Autodesk Inventor part; units mm, degrees
ref_plane "YZ Plane" through (0, 0, 0) normal (1, 0, 0) x (0, 1, 0)
ref_plane "XZ Plane" through (0, 0, 0) normal (0, 1, 0) x (-1, 0, 0)
ref_plane "XY Plane" through (0, 0, 0) normal (0, 0, 1) x (1, 0, 0)
sketch "Sketch1" plane through (0, 0, 0) normal (0, 0, 1) x (1, 0, 0)
  line L0 (0, 0) -> (161.978778, 0)
  line L1 (161.978778, -12.7) -> (0, -12.7)
  line L2 (0, 0) -> (35.7378, 0)
  line L3 (35.7378, 0) -> (35.7378, -1.5875)
  line L4 (35.7378, -1.5875) -> (36.53155, -1.5875)
  line L5 (36.53155, -1.5875) -> (36.53155, 0)
  line L6 (35.7378, -1.5875) -> (34.94405, -1.5875)
  line L7 (34.94405, -1.5875) -> (34.94405, 0)
  line L8 (36.53155, -12.7) -> (34.94405, -12.7)
  line L9 (34.94405, -12.7) -> (34.94405, -11.1125)
  line L10 (34.94405, -11.1125) -> (36.53155, -11.1125)
  line L11 (36.53155, -11.1125) -> (36.53155, -12.7)
  line L12 (161.978778, 0) -> (151.640978, 0)
sketch "Sketch3" plane through (0, 0, 0) normal (0, 0, -1) x (-1, 0, 0)
  circle A0 centre (6.35164, 38.1) radius 3.3782
  circle A1 centre (6.35164, 22.225) radius 3.3782
sketch "Sketch6" plane through (-12.7, 33.655, 84.38515) normal (0, 0, 1) x (1, 0, 0)
  line L0 (0, 0) -> (12.7, 0)
  line L1 (0, -33.655) -> (0, 0)
  line L2 (6.35, 0) -> (6.35, -11.218333)
  line L3 (6.35, -11.218333) -> (6.35, -22.445133)
  circle A0 centre (6.35, -11.218333) radius 3.3782
  circle A1 centre (6.35, -22.445133) radius 3.3782
  dimension "d29" = 11.21833
  dimension "d31" = 11.2268
  dimension "d32" = 6.7564
  dimension "d33" = 6.7564
sketch "Sketch1 outline for Plate1" plane through (0, 0, 0) normal (0, 0, 1) x (1, 0, 0)
  line L0 (0, 0) -> (-12.7, 0)
  line L1 (-12.7, 0) -> (-12.7, 44.45)
  line L2 (-12.7, 44.45) -> (0, 44.45)
  line L3 (0, 44.45) -> (0, 0)
extrude "Plate1" add sketch "Sketch1 outline for Plate1" along normal blind 3.175
sketch "Sketch2" plane through (0, -12.7, 0) normal (0, 0, 1) x (1, 0, 0)
  line L0 (35.7378, 11.1125) -> (35.7378, 12.7)
  line L1 (0, 12.7) -> (35.7378, 12.7)
  line L2 (36.53155, 12.7) -> (161.978778, 12.7)
  line L3 (35.7378, 11.1125) -> (34.94405, 11.1125)
  line L4 (34.94405, 11.1125) -> (34.94405, 12.7)
edge flange "Flange1" height 79.94015 angle 90 thickness 3.175 bend radius 1.27 thickness toward (0, -1, 0) relief straight relief width 3.175 relief depth 1.5875 edges at (-6.35, 0, 3.175) wall of the first edge with corners at (-12.7, -1.27, 4.445) (0, -1.27, 4.445) (0, -1.27, 79.94015) (-12.7, -1.27, 79.94015)
bend "Bend1"
corner "Corner1"
sketch "Sketch4" plane through (0, -12.7, 0) normal (0, 0, 1) x (1, 0, 0)
  line L0 (161.978778, 0) -> (36.53155, 0)
  line L1 (36.53155, 12.7) -> (161.978778, 12.7)
  line L2 (161.978778, 12.7) -> (115.445978, 12.7)
  line L3 (115.445978, 12.7) -> (115.445978, 11.1125)
  line L4 (115.445978, 11.1125) -> (116.239728, 11.1125)
  line L5 (116.239728, 11.1125) -> (116.239728, 12.7)
  line L6 (115.445978, 11.1125) -> (114.652228, 11.1125)
  line L7 (114.652228, 11.1125) -> (114.652228, 12.7)
  line L8 (140.845978, 0) -> (141.639728, 0)
  line L9 (141.639728, 0) -> (141.639728, 1.5875)
  line L10 (141.639728, 1.5875) -> (140.052228, 1.5875)
  line L11 (140.052228, 1.5875) -> (140.052228, 0)
  dimension "d15" = 1.5875
extrude "Cut1" cut sketch "Sketch3" against normal blind 3.175
sketch "Sketch5" plane through (0, -12.7, 0) normal (0, 0, 1) x (1, 0, 0)
  line L0 (115.445978, 12.7) -> (115.445978, 11.1125)
  line L1 (115.445978, 12.7) -> (161.978778, 12.7)
  line L2 (115.445978, 11.1125) -> (116.239728, 11.1125)
  line L3 (116.239728, 11.1125) -> (116.239728, 12.7)
edge flange "Flange2" height 38.1 angle 90 thickness 3.175 bend radius 1.27 thickness toward (0, 0, 1) relief straight relief width 3.175 relief depth 1.5875 edges at (-6.35, -1.27, 79.94015) wall of the first edge with corners at (-12.7, 0, 81.21015) (0, 0, 81.21015) (0, 33.655, 81.21015) (-12.7, 33.655, 81.21015)
bend "Bend2"
corner "Corner2"
extrude "Cut3" cut sketch "Sketch6" against normal blind 3.175
equation "\"d3\" = BendReliefWidth"
equation "\"d4\" = BendReliefDepth"
equation "\"d5\" = MinimumRemnant"
equation "\"d6\" = BendRadius"
equation "\"d10\" = CornerReliefSize"
equation "\"d11\" = GapSize"
equation "\"d12\" = JacobiRadiusSize"
equation "\"d19\" = BendReliefWidth"
equation "\"d20\" = BendReliefDepth"
equation "\"d21\" = MinimumRemnant"
equation "\"d22\" = BendRadius"
equation "\"d26\" = CornerReliefSize"
equation "\"d27\" = GapSize"
equation "\"d28\" = JacobiRadiusSize"
equation "\"BendRadius\" = Thickness"
equation "\"BendReliefWidth\" = Thickness"
equation "\"BendReliefDepth\" = 0.5 * Thickness"
equation "\"CornerReliefSize\" = 4 * Thickness"
equation "\"MinimumRemnant\" = 2 * Thickness"
equation "\"TransitionRadius\" = BendRadius"
equation "\"JacobiRadiusSize\" = Thickness"
equation "\"GapSize\" = Thickness"
equation "\"d2\" = BendRadius"
equation "\"d6\" = Thickness"
equation "\"d16\" = Thickness"
properties part number "M - bottom pulley mount v2" material "Aluminum 6061"
Read the model definition and answer for the solid it produces. Units are mm, in the model's axes. A direction names the side the tool comes from. Coordinates: 2 decimals unless noted, no trailing zeros. Order: outer loops, then holes, each group sorted by start corner. A loop starts at its lowest first (then second) coordinate and runs counter-clockwise, first axis right, second up. Notation, with made-up numbers: (-23.75, 66.5) - (-13.75, 66.5) arc R21 ccw to (-13.75, 98.5) - close; hole circle Ø7 at (24.5, 1). An arc over 180 degrees is marked (long way). Answer as a JSON object with one key per item and string values. Group by question number.
Item 1: Flat-ended cylindrical pins translate along their axes: P1, Ø5.5, axis at x = -6.35, y = 38.1, coming from the -Z side; P2, Ø3, axis at x = -8.5, z = 16.5, coming from the +Y side; P3, Ø1.6, axis at x = -4, z = 83, coming from the +Y side (3 decimals). Find the tip coordinate at first contact, or state that the pin passes through.
Item 2: Section A-A (x = -6.35) is taken. Give the vertices of the cut face in (y, z) (3 decimals), plus the area to 3 significant figures.
Item 3: A tool of negligible diameter and unlimited length cuts with its end or side. For faces 4 (the face through (-6, 33.655, 83)), 5 (the face through (-6, 18, 3.175)), 6 (the face through (-4.79, 19.44, 82.82)), from which of +Z, -Z, +X, -X, +Y, -Y can it reach the whole face along a straight path? Write none if from no direction.
Item 4: Section D-D (x = -11.25) is taken. Give the vertices of the cut face in (y, z) (3 decimals).
Item 5: Section C-C (y = 13) is taken. Give the vertices of the cut face in (x, z) (3 decimals), plus the area to 3 significant figures.
Item 6: The mould has two halves that part along Z. Classify faces 1 (the face through (-6.261, -3.108, 83.118)), 2 (the face through (-6, 17, 81.21)), 3 (the face through (-3.229, 9.916, 82.82)): +Z half, -Z half, draft (parallel to the pull), parting line (faces both ways), or undercut.
Item 7: Section B-B (y = 36) is taken. Give the vertices of the cut face in (x, z) (3 decimals), plus the area to 3 significant figures.
Item 8: Consider probe 1 along Z at (x, y) = (-3.25, 31.5) (3 decimals); probe 2 along Y at (x, z) = (-6.35, 83.3) (3 decimals); probe 3 along Y at (x, z) = (-6.35, 83.2) (3 decimals). Determine where each line is inside the solid, lowest interval first. Write a range as from..to.
Results are:
{
 "1": {"P1": "passes through", "P2": "stops at y = -1.27", "P3": "stops at y = 33.655"},
 "2": {"outline": "(-4.445, 4.445) arc R4.445 ccw to (0, 0) - (18.847, 0) - (18.847, 3.175) - (0, 3.175) arc R1.27 cw to (-1.27, 4.445) - (-1.27, 79.94) arc R1.27 cw to (0, 81.21) - (7.832, 81.21) - (7.832, 84.385) - (0, 84.385) arc R4.445 ccw to (-4.445, 79.94) - close; (14.588, 81.21) - (19.058, 81.21) - (19.058, 84.385) - (14.588, 84.385) - close; (25.603, 0) - (34.722, 0) - (34.722, 3.175) - (25.603, 3.175) - close; (25.815, 81.21) - (33.655, 81.21) - (33.655, 84.385) - (25.815, 84.385) - close; (41.478, 0) - (44.45, 0) - (44.45, 3.175) - (41.478, 3.175) - close", "area": "430 mm^2"},
 "3": {"face 4": "+Z, +X, -X, +Y", "face 5": "+X, -X, +Y", "face 6": "+Z"},
 "4": {"outline": "(-4.445, 4.445) arc R4.445 ccw to (0, 0) - (44.45, 0) - (44.45, 3.175) - (0, 3.175) arc R1.27 cw to (-1.27, 4.445) - (-1.27, 79.94) arc R1.27 cw to (0, 81.21) - (33.655, 81.21) - (33.655, 84.385) - (0, 84.385) arc R4.445 ccw to (-4.445, 79.94) - close"},
 "5": {"outline": "(-12.7, 0) - (0, 0) - (0, 3.175) - (-12.7, 3.175) - close; (-12.7, 81.21) - (-9.215, 81.21) - (-9.215, 84.385) - (-12.7, 84.385) - close; (-3.485, 81.21) - (0, 81.21) - (0, 84.385) - (-3.485, 84.385) - close", "area": "62.5 mm^2"},
 "6": {"face 1": "+Z half", "face 2": "undercut", "face 3": "draft"},
 "7": {"outline": "(-12.7, 0) - (-8.998, 0) - (-8.998, 3.175) - (-12.7, 3.175) - close; (-3.705, 0) - (0, 0) - (0, 3.175) - (-3.705, 3.175) - close", "area": "23.5 mm^2"},
 "8": {"probe 1": "z = 0..3.175, 81.21..84.385", "probe 2": "y = -2.91..7.832, 14.588..19.058, 25.815..33.655", "probe 3": "y = -3.022..7.832, 14.588..19.058, 25.815..33.655"}
}
